Verification items for the finished model (mm, model axes). A direction names the side the tool comes from. Coordinates: 2 decimals unless noted, no trailing zeros. Write each loop counter-clockwise with the first axis right and the second up, starting at its lowest first coordinate (ties: lowest second). Pieces come first, ordered by that corner, then holes. Notation, with made-up numbers: (56, 9.25) - (69, 9.25) arc R23 cw to (69, 23.25) - close; hole circle Ø8 at (61.25, -35). An arc over 180 degrees is marked (long way). Answer as CSV lines item,"result". Start each with the question number.
```python
from build123d import *

# Parameters (mm, degrees)
BOSS_EXTRUDE1_DEPTH = 3.175
SKETCH2_W           = 9.525
SKETCH2_H           = 6.35
BOSS_EXTRUDE2_DEPTH = 6.35
CUT_EXTRUDE1_DEPTH  = 78.291604858


with BuildPart() as part:
    # Sketch1 → Boss-Extrude1 (new, symmetric)
    with BuildSketch(Plane(origin=(0, 0, 0), x_dir=(1, 0, 0), z_dir=(0, 1, 0))):
        with BuildLine():
            Line((-41.502443258, -43.180856192), (-54.202443258, -43.180856192))
            ThreePointArc((-54.202443258, -43.180856192), (-28.976499653, -54.667950949), (-5.512754363, -39.911452934))
            ThreePointArc((-5.512754363, -39.911452934), (-14.460289915, -46.180199356), (-24.965503608, -43.180856192))
            Line((-24.965503608, -43.180856192), (-41.502443258, -43.180856192))
        make_face()
    extrude(amount=BOSS_EXTRUDE1_DEPTH, both=True)

    # Sketch2 → Boss-Extrude2 (add)
    with BuildSketch(Plane(origin=(0, 3.175, 0), x_dir=(1, 0, 0), z_dir=(0, 1, 0))):
        with Locations((-39.583973433, -40.005856192)):
            Rectangle(SKETCH2_W, SKETCH2_H)
    extrude(amount=-BOSS_EXTRUDE2_DEPTH)

    # Sketch3 → Cut-Extrude1 (cut, through all)
    with BuildSketch(Plane(origin=(0, 3.175, 0), x_dir=(1, 0, 0), z_dir=(0, 1, 0))):
        with BuildLine():
            ThreePointArc((-5.512754363, -39.911452934), (-7.527252939, -42.578004595), (-10.167597026, -44.626732342))
            ThreePointArc((-10.167597026, -44.626732342), (-9.515060164, -44.74815939), (-9.539624144, -45.411443263))
            ThreePointArc((-9.539624144, -45.411443263), (-7.365201872, -42.779316528), (-5.512754363, -39.911452934))
        make_face()
    extrude(amount=-CUT_EXTRUDE1_DEPTH, mode=Mode.SUBTRACT)


solid = part.part
```
1. Cross-section at B-B (z = 40). Record the cut outline in (x, y) (3 decimals), and give its area (3 significant figures).
2. Access from +Z, -Z, +X, -X, +Y, -Y to the whole of each face (thin tool, end or side, straight path). Record for faces 1 (the face through (-34.821, 0, 40)), 2 (the face through (-49, 0, 43.181)), 3 (the face through (-17.69, 0.044, 46.306)).
3. Draft check along X on faces 4 (the face through (-40, 0, 36.831)), 5 (the face through (-44.346, 0, 40)), 6 (the face through (-9.52, 0.04, 44.74)). Enter one of: pulls with the +X half, pulls with the -X half, needs draft (parallel to the pull), parting line crosses it, or undercut.
4. Depth check by flat-ended pin: P1, Ø3, axis at y = -0.5, z = 52, coming from the -X side; P2, Ø3, axis at y = 0, z = 40.5, coming from the +X side. Enter the tip coordinate at first touch or a pass-through.
5. Cross-section at A-A (y = 1.75). Record the cut outline in (x, z), and give its area (3 significant figures).
6. Cross-section at C-C (x = -23.5). Record the cut outline in (y, z) (3 decimals), and give its area (3 significant figures).
7. Scan lines: line 1 along X through (y, z) = (0.75, 40.5); line 2 along Z through (x, y) = (-31, 0.75); line 3 along Z through (x, y) = (-49, -0.25). Record each from-to range of solid material in increasing order. Write a range as from..to.
Completed:
1,outline,"(-44.346, -3.175) - (-34.821, -3.175) - (-34.821, 3.175) - (-44.346, 3.175) - close"
1,area,"60.5 mm2"
2,face 1,"-Z, +X, +Y, -Y"
2,face 2,"-Z, -X, +Y, -Y"
2,face 3,"-Z, +Y, -Y"
3,face 4,"needs draft"
3,face 5,"pulls with the -X half"
3,face 6,"undercut"
4,P1,"stops at x = -46.08"
4,P2,"stops at x = -34.82"
5,outline,"(-54.2, 43.18) - (-44.35, 43.18) - (-44.35, 36.83) - (-34.82, 36.83) - (-34.82, 43.18) - (-24.97, 43.18) arc R12.7 cw to (-10.17, 44.63) arc R0.51 ccw to (-9.54, 45.41) arc R29.21 ccw to start"
5,area,"398 mm2"
6,outline,"(-3.175, 44.295) - (3.175, 44.295) - (3.175, 53.772) - (-3.175, 53.772) - close"
6,area,"60.2 mm2"
7,line 1,"x = -44.35..-34.82"
7,line 2,"z = 43.18..54.73"
7,line 3,"z = 43.18..48.48"
